```python
from build123d import *

# Parameters (mm, degrees)
SKETCH1_R           = 12.5
BOSS_EXTRUDE1_DEPTH = 8
SKETCH2_R           = 6
CUT_EXTRUDE1_DEPTH  = 20.403607912
SKETCH3_W           = 4
SKETCH3_H           = 4
CUT_EXTRUDE2_DEPTH  = 20.403607912
CHAMFER1_SIZE       = 1


with BuildPart() as part:
    # Sketch1 → Boss-Extrude1 (new body)
    with BuildSketch(Plane.XY):
        Circle(SKETCH1_R)
    extrude(amount=BOSS_EXTRUDE1_DEPTH)

    # Sketch2 → Cut-Extrude1 (cut, through all)
    with BuildSketch(Plane.XY.offset(8)):
        Circle(SKETCH2_R)
    extrude(amount=-CUT_EXTRUDE1_DEPTH, mode=Mode.SUBTRACT)

    # Sketch3 → Cut-Extrude2 (cut, through all)
    with BuildSketch(Plane.XY.offset(8)):
        with Locations((12.5, 0)):
            Rectangle(SKETCH3_W, SKETCH3_H)
        with Locations((0, 12.5)):
            Rectangle(SKETCH3_W, SKETCH3_H)
        with Locations((0, -12.5)):
            Rectangle(SKETCH3_W, SKETCH3_H)
        with Locations((-12.5, 0)):
            Rectangle(SKETCH3_W, SKETCH3_H)
    extrude(amount=-CUT_EXTRUDE2_DEPTH, mode=Mode.SUBTRACT)

    # Chamfer1
    chamfer1_edges = [part.edges().sort_by_distance(p)[0] for p in [
        (-8.838834765, 8.838834765, 8),
        (-8.838834765, -8.838834765, 8),
        (8.838834765, -8.838834765, 8),
        (8.838834765, 8.838834765, 8),
    ]]
    chamfer(chamfer1_edges, length=CHAMFER1_SIZE)


solid = part.part
```
Read the model definition and answer for the solid it produces. Units are mm, in the model's axes. A direction names the side the tool comes from. Round coordinates to 2 decimals unless told otherwise and drop trailing zeros. Loops run counter-clockwise (first coordinate to the right, second up) from the corner with the lowest first, then second, coordinate; pieces in that order, holes last. Notation, with made-up numbers: (25.25, 85.25) -> (79.25, 85.25) arc R20 ccw to (79.25, 90.25) -> close; hole circle Ø8 at (-12, 65.25). An arc over 180 degrees is marked (long way). One line per item, written item: value.
1) For faces 5 (the face through (-6, 0, 4)), 6 (the face through (-11, 2, 4)), 7 (the face through (11, 2, 4)), 8 (the face through (2, -11, 4)), 9 (the face through (2, 11, 4)), determine the directions among +Z, -Z, +X, -X, +Y, -Y from which every point of the face is accessible in a straight line to the end or side of a thin tool.
Answer list:
face 5: +Z, -Z
face 6: +Z, -Z, -X
face 7: +Z, -Z, +X
face 8: +Z, -Z, -Y
face 9: +Z, -Z, +Y
2) Flat-ended cylindrical pins translate along their axes: P1, Ø12, axis at x = 8.5, y = 5, coming from the -Z side; P2, Ø1.5, axis at y = 12, z = 5, coming from the -X side; P3, Ø2, axis at x = 0.5, z = 2.5, coming from the +Y side; P4, Ø2, axis at x = -11.5, z = 3, coming from the -Y side. Find the tip coordinate at first contact, or state that the pin passes through.
Answer list:
P1: stops at z = 0
P2: stops at x = -5.45
P3: stops at y = 10.5
P4: stops at y = -6.78
3) A cutting plane is placed at B-B (z = 6.25). Determine the outline of the cut face in (x, y), and give its area (3 significant figures).
Answer list:
outline: (-12.34, -2) arc R12.5 ccw to (-2, -12.34) -> (-2, -10.5) -> (2, -10.5) -> (2, -12.34) arc R12.5 ccw to (12.34, -2) -> (10.5, -2) -> (10.5, 2) -> (12.34, 2) arc R12.5 ccw to (2, 12.34) -> (2, 10.5) -> (-2, 10.5) -> (-2, 12.34) arc R12.5 ccw to (-12.34, 2) -> (-10.5, 2) -> (-10.5, -2) -> close; hole circle Ø12 at (0, 0)
area: 347 mm²
4) The mould has two halves that part along X. Classify faces 1 (the face through (11, -2, 4)), 2 (the face through (-10.5, 0, 4)), 3 (the face through (-2, 11, 4)), 4 (the face through (8.32, 8.17, 7.84)): pulls with the +X half, pulls with the -X half, needs draft (parallel to the pull), parting line crosses it, or undercut.
Answer list:
face 1: needs draft
face 2: pulls with the -X half
face 3: undercut
face 4: pulls with the +X half
5) Consider L1, parallel to Y at x = 0, z = 6; L2, parallel to X at y = 2.25, z = 4; L3, parallel to X at y = 3.5, z = 2.5. Determine where each line is inside the solid, lowest interval first. Write a range as [from, to].
Answer list:
L1: y = [-10.5, -6], [6, 10.5]
L2: x = [-12.3, -5.56], [5.56, 12.3]
L3: x = [-12, -4.87], [4.87, 12]
6) A cutting plane is placed at A-A (y = 0). Determine the outline of the cut face in (x, z), and give its area (3 significant figures).
Answer list:
outline: (-10.5, 0) -> (-6, 0) -> (-6, 8) -> (-10.5, 8) -> close; (6, 0) -> (10.5, 0) -> (10.5, 8) -> (6, 8) -> close
area: 72.0 mm²
